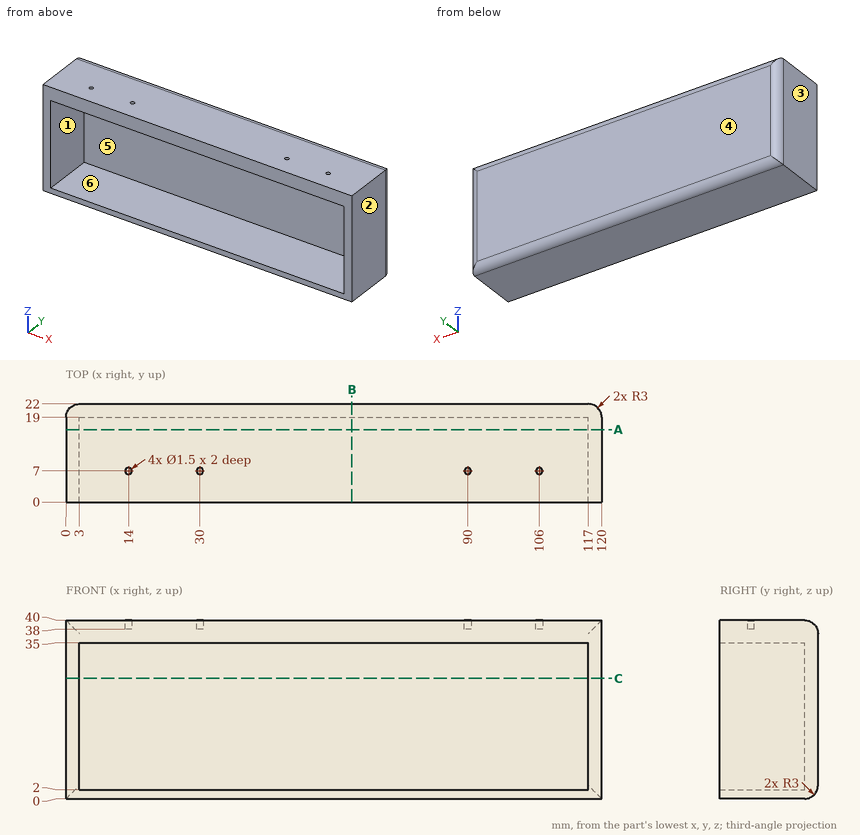
Job drawing, mm, ordinate dimensions from the low corner. One solid piece. A direction names the side the tool comes from. Coordinates: 2 decimals unless noted, no trailing zeros. Order: outer loops, then holes, each group sorted by start corner. A loop starts at its lowest first (then second) coordinate and runs counter-clockwise, first axis right, second up. Notation, with made-up numbers: (-40, -39) - (6, -39) arc R15 cw to (6, -10) - close; hole circle Ø3 at (58, -10.75). An arc over 180 degrees is marked (long way). Use CSV: the item, a comma, the result in double quotes.
Item 1: Saw through at B-B on x = 64. Give the cut face in (y, z), and give its area (3 significant figures).
Solved:
outline,"(0, 0) - (19, 0) arc R3 ccw to (22, 3) - (22, 37) arc R3 ccw to (19, 40) - (0, 40) - (0, 35) - (19, 35) - (19, 2) - (0, 2) - close"
area,"249 mm²"
Item 2: Drop flat-ended pins along their axis: P1, Ø0.9, axis at x = 90, y = 7, coming from the +Z side; P2, Ø2, axis at x = 17.5, z = 26.5, coming from the -Y side. Give the stop position or say it passes through.
Solved:
P1,"stops at z = 38"
P2,"stops at y = 19"
Item 3: Saw through at A-A on y = 16.25. Give the cut face in (x, z).
Solved:
outline,"(0, 0) - (120, 0) - (120, 40) - (0, 40) - close; hole (3, 2) - (117, 2) - (117, 35) - (3, 35) - close"
Item 4: Saw through at C-C on z = 27. Give the cut face in (x, y), and give its area (3 significant figures).
Solved:
outline,"(0, 0) - (3, 0) - (3, 19) - (117, 19) - (117, 0) - (120, 0) - (120, 19) arc R3 ccw to (117, 22) - (3, 22) arc R3 ccw to (0, 19) - close"
area,"470 mm²"
Item 5: Mould opens along X. For the marked faces 3, 4, 5 and 6 say: +X half, -X half, draft (parallel to the pull), parting line (faces both ways), or undercut.
Solved:
face 3,"-X half"
face 4,"draft"
face 5,"undercut"
face 6,"undercut"
Item 6: Probe probe 1 along Z at (x, y) = (71.5, 4.25); probe 2 along X at (y, z) = (2.75, 21.5); probe 3 along Y at (x, z) = (106, 39). List the from-to ranges inside material, lowest first.
Solved:
probe 1,"z = 0 to 2, 35 to 40"
probe 2,"x = 0 to 3, 117 to 120"
probe 3,"y = 0 to 6.25, 7.75 to 21.24"
Item 7: 3-axis set-ups, long thin cutter, end or side, ignore diameter. For the marked faces 1 and 2: which of +Z, -Z, +X, -X, +Y, -Y reach the whole face in a straight line?
Solved:
face 1,"-Y"
face 2,"+Z, -Z, +X, +Y, -Y"
